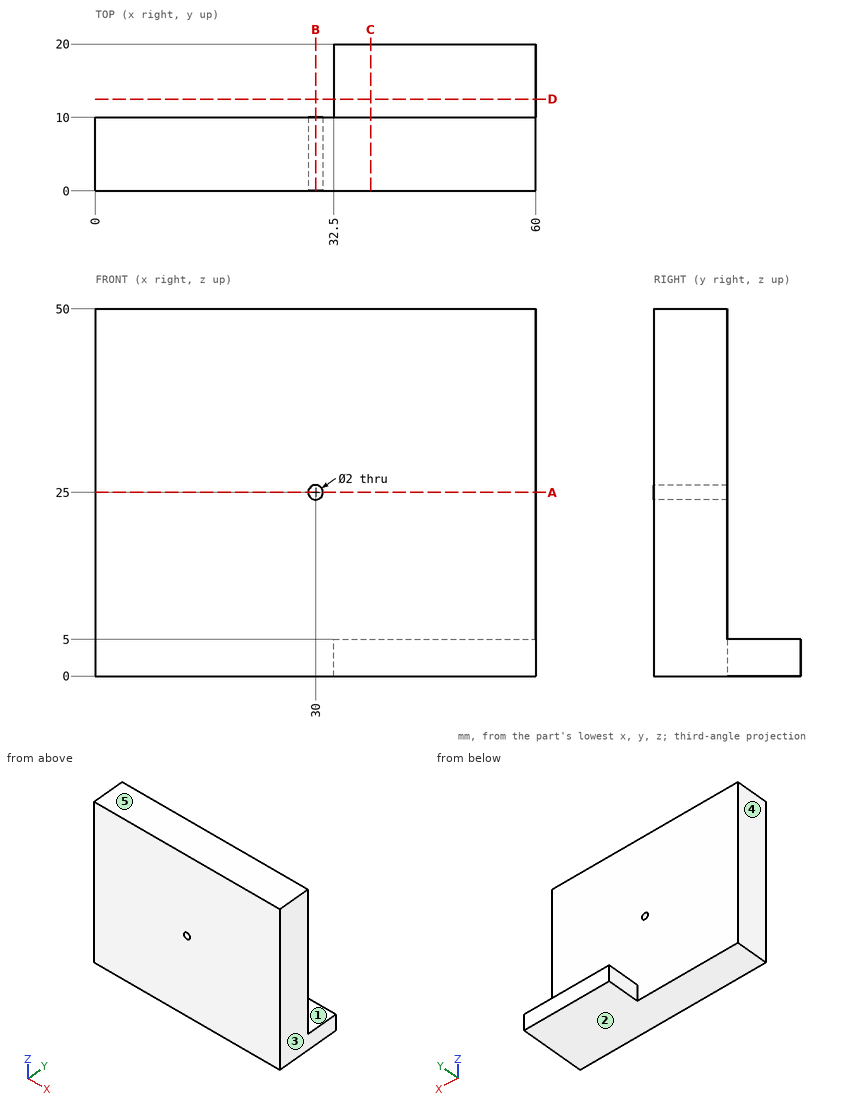
The drawing under review shows one solid part. Ordinate dimensions are in mm from its lowest x, y, z. A direction names the side the tool comes from. Round coordinates to 2 decimals unless told otherwise and drop trailing zeros. Order: outer loops, then holes, each group sorted by start corner. A loop starts at its lowest first (then second) coordinate and runs counter-clockwise, first axis right, second up. Notation, with made-up numbers: (31, 41.5) - (66, 41.5) arc R16 ccw to (66, 50.5) - close; hole circle Ø9 at (5.25, -6). An arc over 180 degrees is marked (long way). Return JSON: item names as keys, results as strings.
Q1. The part is to be moulded in two halves that separate along X. For the marked faces 3, 4 and 5, say which applies: pulls with the +X half, pulls with the -X half, needs draft (parallel to the pull), parting line crosses it, or undercut.
Computed values:
{"face 3": "pulls with the +X half", "face 4": "pulls with the -X half", "face 5": "needs draft"}
Q2. Machinability: for the marked faces 1 and 2, which of the approach directions +Z, -Z, +X, -X, +Y, -Y give a long, thin tool a straight path to every point of the face, cutting with its end or side? Answer none if there is none.
Computed values:
{"face 1": "+Z, +X, -X, +Y", "face 2": "-Z, +X, -X, +Y, -Y"}
Q3. Consider section B-B on x = 30. Write out the cut boundary in (y, z), plus the area to 3 significant figures.
Computed values:
{"outline": "(0, 0) - (10, 0) - (10, 24) - (0, 24) - close; (0, 26) - (10, 26) - (10, 50) - (0, 50) - close", "area": "480 mm2"}
Q4. For pin 1 Ø15 at (x, z) = (31.5, 26) entering from +Y; pin 2 Ø1.8 at (x, z) = (30, 25) entering from +Y; pin 3 Ø8 at (x, y) = (41, 16.5) entering from +Z; pin 4 Ø1.5 at (y, z) = (17, 1.5) entering from -X, all flat-tipped, find the tip position at first contact; note any pin that passes through.
Computed values:
{"pin 1": "stops at y = 10", "pin 2": "passes through", "pin 3": "stops at z = 5", "pin 4": "stops at x = 32.5"}
Q5. Consider section A-A on z = 25. Write out the cut boundary in (x, y).
Computed values:
{"outline": "(0, 0) - (29, 0) - (29, 10) - (0, 10) - close; (31, 0) - (60, 0) - (60, 10) - (31, 10) - close"}
Q6. Wall thickness on L1, parallel to X at y = 5.5, z = 25; L2, parallel to Z at x = 30, y = 3; L3, parallel to Y at x = 8, z = 9.5: over which ranges is each line inside the solid? List them lowest first. Write a range as [from, to].
Computed values:
{"L1": "x = [0, 29], [31, 60]", "L2": "z = [0, 24], [26, 50]", "L3": "y = [0, 10]"}
Q7. Consider section C-C on x = 37.5. Write out the cut boundary in (y, z), plus the area to 3 significant figures.
Computed values:
{"outline": "(0, 0) - (20, 0) - (20, 5) - (10, 5) - (10, 50) - (0, 50) - close", "area": "550 mm2"}
Q8. Consider section D-D on y = 12.5. Write out the cut boundary in (x, z), plus the area to 4 significant figures.
Computed values:
{"outline": "(32.5, 0) - (60, 0) - (60, 5) - (32.5, 5) - close", "area": "137.5 mm2"}
